from build123d import *

# Parameters (mm, degrees)
F1_DEPTH = 6
F2_R     = 9.5
F3_DEPTH = 7
F4_R     = 2
F5_R     = 1


with BuildPart() as f1:
    # F0 (on Top) → F1 (new body)
    with BuildSketch(Plane.XY):
        Polygon((-8.198368, 10.017881), (-10, 5.773503), (-5, 8.660254), align=None)
        with BuildLine():
            ThreePointArc((-10, 5.773503), (-12, 2.886751), (-10, 0))
            Line((-10, 0), (-10, 5.773503))
        make_face()
        with BuildLine():
            ThreePointArc((-10, 0), (-12, -2.886751), (-10, -5.773503))
            Line((-10, -5.773503), (-10, 0))
        make_face()
        Polygon((-4.576555, 12.108936), (-5, 8.660254), (0, 11.547005), align=None)
        Polygon((4.576555, 12.108936), (0, 11.547005), (5, 8.660254), align=None)
        Polygon((0, -11.547005), (-5, -8.660254), (-4.576555, -12.108936), align=None)
        Polygon((8.198368, 10.017881), (5, 8.660254), (10, 5.773503), align=None)
        with BuildLine():
            Line((10, 0), (10, -5.773503))
            ThreePointArc((10, -5.773503), (12, -2.886751), (10, 0))
        make_face()
        with BuildLine():
            Line((10, 5.773503), (10, 0))
            ThreePointArc((10, 0), (12, 2.886751), (10, 5.773503))
        make_face()
        Polygon((-5, -8.660254), (-10, -5.773503), (-8.198368, -10.017881), align=None)
        Polygon((5, -8.660254), (0, -11.547005), (4.576555, -12.108936), align=None)
        Polygon((10, -5.773503), (5, -8.660254), (8.198368, -10.017881), align=None)
        Polygon((-10, 0), (-10, -5.773503), (-5, -8.660254), (0, -11.547005), (5, -8.660254), (10, -5.773503), (10, 0), (10, 5.773503), (5, 8.660254), (0, 11.547005), (-5, 8.660254), (-10, 5.773503), align=None)
    extrude(amount=F1_DEPTH)

    # F2 (on face) → F3 (cut)
    with BuildSketch(Plane(origin=(0, 0, 0), x_dir=(1, 0, 0), z_dir=(0, 0, -1))):
        Circle(F2_R)
    extrude(amount=-F3_DEPTH, mode=Mode.SUBTRACT)

    # F4
    f4_edges = [f1.edges().sort_by_distance(p)[0] for p in [
        (5, 8.660254, 3),
        (-5, 8.660254, 3),
        (5, -8.660254, 3),
        (-5, -8.660254, 3),
        (10, 0, 3),
        (-10, 0, 3),
    ]]
    fillet(f4_edges, radius=F4_R)

    # F5
    f5_edges = [f1.edges().sort_by_distance(p)[0] for p in [
        (-9.5, 0, 6),
        (-9.5, 0, 0),
    ]]
    fillet(f5_edges, radius=F5_R)


solid = f1.part
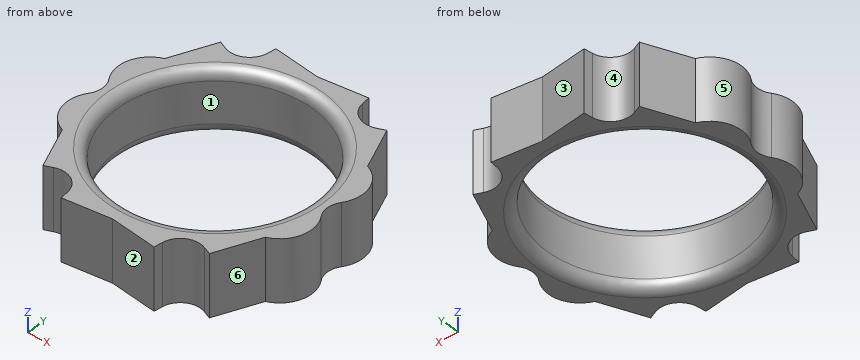
CAD build for the part. Positions are in the model's coordinates, mm. Face numbers are marked on the shaded views. A direction names the side the tool comes from. Round coordinates to 2 decimals unless told otherwise and drop trailing zeros. Return JSON: item names as keys, results as strings.
(1) Tool access for the marked faces 1, 2 and 3: list every direction of +Z, -Z, +X, -X, +Y, -Y with a clear straight run to the whole face (end or side of a thin tool).
Answer key:
{"face 1": "+Z, -Z", "face 2": "+Z, -Z, -Y", "face 3": "+Z, -Z, +Y"}
(2) Pin check, flat tips, straight feed: pin 1 Ø2 at (y, z) = (6.5, 4.5) entering from +X; pin 2 Ø5 at (x, y) = (6, -4.5) entering from -Z. Stop position of each tip, or through.
Answer key:
{"pin 1": "stops at x = 10.55", "pin 2": "stops at z = 0.13"}
(3) Pull direction X, two halves, no side cores. Call the marked faces 4, 5 and 6: +X half, -X half, draft (parallel to the pull), parting line (faces both ways), or undercut.
Answer key:
{"face 4": "undercut", "face 5": "-X half", "face 6": "+X half"}
(4) Wall check: probe 1 along Y at (x, z) = (0, 4.05); probe 2 along X at (y, z) = (0, 4.05); probe 3 along Y at (x, z) = (-4.25, 5). Give the ranges that are in metal, low to high. Write a range as from..to.
Answer key:
{"probe 1": "y = -11.55..-9.5, 9.5..11.55", "probe 2": "x = -11.1..-9.5, 9.5..11.1", "probe 3": "y = -12.07..-8.5, 8.5..12.07"}
